Autodesk Inventor part; units mm, degrees
ref_plane "Startebene" through (0, 0, 0) normal (0, 0, 1) x (1, 0, 0)
ref_plane "Endebene" through (0, 0, 320) normal (0, 0, 1) x (1, 0, 0)
ref_plane "Startebene1" through (0, 0, 0) normal (0, 0, 1) x (1, 0, 0)
ref_plane "Startebene" through (0, 0, 0) normal (0, 0, 1) x (1, 0, 0)
ref_plane "Endebene" through (0, 0, 320) normal (0, 0, 1) x (1, 0, 0)
ref_plane "Startebene1" through (0, 0, 0) normal (0, 0, 1) x (1, 0, 0)
ref_plane "Endebene1" through (0, 0, 40) normal (0, 0, 1) x (1, 0, 0)
ref_plane "Startebene2" through (0, 0, 0) normal (0, 0, 1) x (1, 0, 0)
ref_plane "Endebene2" through (0, 0, 40) normal (0, 0, 1) x (1, 0, 0)
ref_plane "Startebene3" through (0, 0, 0) normal (0, 0, 1) x (1, 0, 0)
ref_plane "Endebene3" through (0, 0, 160) normal (0, 0, 1) x (1, 0, 0)
sketch "Skizze" plane through (0, 0, 0) normal (0, 0, 1) x (1, 0, 0)
  line L0 (-10, 9) -> (-10, 3.3)
  arc A0 (-10, 3.3) -> (-9.7, 3) centre (-9.7, 3.3) ccw
  line L1 (-9.7, 3) -> (-8, 3)
  line L2 (-8, 3) -> (-8, 6)
  line L3 (-8, 6) -> (-7.0607, 6)
  line L4 (-7.0607, 6) -> (-4, 2.9393)
  line L5 (-4, 2.9393) -> (-4, 0.3)
  line L6 (-4, 0.3) -> (-3.7, 0)
  line L7 (-3.7, 0) -> (-4, -0.3)
  line L8 (-4, -0.3) -> (-4, -2.9393)
  line L9 (-4, -2.9393) -> (-7.0607, -6)
  line L10 (-7.0607, -6) -> (-8, -6)
  line L11 (-8, -6) -> (-8, -3)
  line L12 (-8, -3) -> (-9.7, -3)
  arc A1 (-9.7, -3) -> (-10, -3.3) centre (-9.7, -3.3) ccw
  line L13 (-10, -3.3) -> (-10, -9)
  arc A2 (-10, -9) -> (-9, -10) centre (-9, -9) ccw
  line L14 (-9, -10) -> (-3.3, -10)
  arc A3 (-3.3, -10) -> (-3, -9.7) centre (-3.3, -9.7) ccw
  line L15 (-3, -9.7) -> (-3, -8)
  line L16 (-3, -8) -> (-6, -8)
  line L17 (-6, -8) -> (-6, -7.0607)
  line L18 (-6, -7.0607) -> (-2.9393, -4)
  line L19 (-2.9393, -4) -> (-0.3, -4)
  line L20 (-0.3, -4) -> (0, -3.7)
  line L21 (0, -3.7) -> (0.3, -4)
  line L22 (0.3, -4) -> (2.9393, -4)
  line L23 (2.9393, -4) -> (6, -7.0607)
  line L24 (6, -7.0607) -> (6, -8)
  line L25 (6, -8) -> (3, -8)
  line L26 (3, -8) -> (3, -9.7)
  arc A4 (3, -9.7) -> (3.3, -10) centre (3.3, -9.7) ccw
  line L27 (3.3, -10) -> (9, -10)
  arc A5 (9, -10) -> (10, -9) centre (9, -9) ccw
  line L28 (10, -9) -> (10, -3.3)
  arc A6 (10, -3.3) -> (9.7, -3) centre (9.7, -3.3) ccw
  line L29 (9.7, -3) -> (8, -3)
  line L30 (8, -3) -> (8, -6)
  line L31 (8, -6) -> (7.0607, -6)
  line L32 (7.0607, -6) -> (4, -2.9393)
  line L33 (4, -2.9393) -> (4, -0.3)
  line L34 (4, -0.3) -> (3.7, 0)
  line L35 (3.7, 0) -> (4, 0.3)
  line L36 (4, 0.3) -> (4, 2.9393)
  line L37 (4, 2.9393) -> (7.0607, 6)
  line L38 (7.0607, 6) -> (8, 6)
  line L39 (8, 6) -> (8, 3)
  line L40 (8, 3) -> (9.7, 3)
  arc A7 (9.7, 3) -> (10, 3.3) centre (9.7, 3.3) ccw
  line L41 (10, 3.3) -> (10, 9)
  arc A8 (10, 9) -> (9, 10) centre (9, 9) ccw
  line L42 (9, 10) -> (3.3, 10)
  arc A9 (3.3, 10) -> (3, 9.7) centre (3.3, 9.7) ccw
  line L43 (3, 9.7) -> (3, 8)
  line L44 (3, 8) -> (6, 8)
  line L45 (6, 8) -> (6, 7.0607)
  line L46 (6, 7.0607) -> (2.9393, 4)
  line L47 (2.9393, 4) -> (0.3, 4)
  line L48 (0.3, 4) -> (0, 3.7)
  line L49 (0, 3.7) -> (-0.3, 4)
  line L50 (-0.3, 4) -> (-2.9393, 4)
  line L51 (-2.9393, 4) -> (-6, 7.0607)
  line L52 (-6, 7.0607) -> (-6, 8)
  line L53 (-6, 8) -> (-3, 8)
  line L54 (-3, 8) -> (-3, 9.7)
  arc A10 (-3, 9.7) -> (-3.3, 10) centre (-3.3, 9.7) ccw
  line L55 (-3.3, 10) -> (-9, 10)
  arc A11 (-9, 10) -> (-10, 9) centre (-9, 9) ccw
  circle A12 centre (0, 0) radius 2.75
  dimension "d2" = 5.5
  dimension "d3" = 10
  dimension "d4" = 10
  dimension "d5" = 5.7
  dimension "d6" = 5.7
  dimension "d7" = 1.7
  dimension "d8" = 3
  dimension "d9" = 0.3
  dimension "d10" = 90
  dimension "d11" = 45
  dimension "d12" = 45
  dimension "d13" = 45
  dimension "d14" = 90
  dimension "d15" = 90
  dimension "d16" = 45
  dimension "d17" = 45
  dimension "d18" = 45
  dimension "d19" = 45
  dimension "d20" = 90
  dimension "d21" = 90
  dimension "d22" = 45
  dimension "d23" = 45
  dimension "d24" = 90
  dimension "d25" = 90
  dimension "d26" = 90
  dimension "d27" = 90
  dimension "d28" = 90
  dimension "d29" = 90
  dimension "d30" = 90
  dimension "d31" = 90
  dimension "d32" = 90
  dimension "d33" = 90
  dimension "d34" = 90
  dimension "d35" = 90
  dimension "d36" = 90
  dimension "d37" = 90
  dimension "d38" = 90
  dimension "d39" = 4
  dimension "d40" = 6
  dimension "d41" = 13
  dimension "d42" = 14
  dimension "d43" = 16
  dimension "d44" = 18
  dimension "d45" = 3
  dimension "d46" = 9
  dimension "d47" = 7
  dimension "d48" = 1
  dimension "d49" = 7
  dimension "d50" = 1.5
  dimension "d51" = 1.8663
  dimension "d52" = 3.3663
  dimension "d53" = 1.5
  dimension "d54" = 1.8663
  dimension "d55" = 3.3663
  dimension "d56" = 4
  dimension "d57" = 10.8187
  dimension "d58" = 1.9092
  dimension "d59" = 5
  dimension "d60" = 13
  dimension "d61" = 13
  dimension "d62" = 16.0513
  dimension "d63" = 3.3234
  dimension "d64" = 14
  dimension "d65" = 12.685
extrude "Körper" add sketch "Skizze" along normal up to surface (160 mm away) from surface at 0
sketch "Skizze21" plane through (0, 0, 0) normal (0, 0, 1) x (1, 0, 0)
  line L0 (0, 0) -> (10, 0)
ref_plane "Arbeitsebene18" through (0, 0, 0) normal (0, -1, 0) x (1, 0, 0)
sketch "Skizze22" plane through (0, 0, 0) normal (0, -1, 0) x (1, 0, 0)
  line L0 (-2, 0) -> (12, 0)
  line L1 (-2, 160) -> (12, 160)
  dimension "d80" = 160
equation "\"G_OFFSET_START\" = 0"
equation "\"G_OFFSET_END\" = 0"
equation "\"G_L\" = d80"
equation "\"G_OFFSET_START1\" = 0"
equation "\"G_OFFSET_END1\" = 0"
equation "\"G_OFFSET_START2\" = 0"
equation "\"G_OFFSET_END2\" = 0"
equation "\"G_OFFSET_START3\" = 0"
equation "\"G_OFFSET_END3\" = 0"
properties part number "Alu Profil 20x20 - AP2020"
Geometry check sheet. Reference: the model listing, model coordinates, mm. A direction names the side the tool comes from. Coordinates: 2 decimals unless noted, no trailing zeros. Use one line per item in the form item = value. Start each with the question number.
1) Set-up check for faces 1 (the flat face through (-10, 6, 79)), 2 (the flat face through (-4.45, 5.51, 78.88)), 3 (the flat face through (-6, -10, 79)), 4 (the flat face through (2, 4, 79)), 5 (the flat face through (4, 2, 79)): record each of +Z, -Z, +X, -X, +Y, -Y from which the full face is reachable in a straight line by a thin tool's end or side.
2) Go/stop test with flat-tipped pins: pin 1 Ø1.5 at (x, y) = (1.5, 5) entering from +Z; pin 2 Ø1.3 at (y, z) = (1, 114.5) entering from -X; pin 3 Ø0.8 at (y, z) = (-1.5, 60.5) entering from +X; pin 4 Ø2 at (x, z) = (-1, 27.5) entering from +Y. Record where each tip stops, or that it passes through.
3) Release check for a two-part mould opening along X. For faces 6 (the flat face through (-8, 4, 79)), 7 (the flat face through (-10, -6, 79)), 8 (the flat face through (10, 6, 79)), 9 (the flat face through (-6, 10, 79)) record: pulls with the +X half, pulls with the -X half, needs draft (parallel to the pull), parting line crosses it, or undercut.
4) Thickness scan on probe 1 along X at (y, z) = (-8.25, 40); probe 2 along X at (y, z) = (-5.25, 106); probe 3 along X at (y, z) = (4.25, 152.5). Record the ranges inside material, lowest first. Write a range as from..to.
Responses:
q1.face_1 = +Z, -Z, -X, +Y, -Y
q1.face_2 = +Z, -Z
q1.face_3 = +Z, -Z, +X, -X, -Y
q1.face_4 = +Z, -Z, +Y
q1.face_5 = +Z, -Z, +X
q2.pin_1 = through
q2.pin_2 = -4
q2.pin_3 = 4
q2.pin_4 = 4
q3.face_6 = undercut
q3.face_7 = pulls with the -X half
q3.face_8 = pulls with the +X half
q3.face_9 = needs draft
q4.probe_1 = -10..-3, 3..10
q4.probe_2 = -10..-8, -6.31..-4.19, 4.19..6.31, 8..10
q4.probe_3 = -10..-8, -5.31..-3.19, 3.19..5.31, 8..10
